Verification items for the finished model (mm, model axes). A direction names the side the tool comes from. Round coordinates to 2 decimals unless told otherwise and drop trailing zeros. Write each loop counter-clockwise with the first axis right and the second up, starting at its lowest first coordinate (ties: lowest second). Pieces come first, ordered by that corner, then holes. Notation, with made-up numbers: M 18.25,87 L 48.25,87 A20 cw 48.25,113 Z; hole C 11,62.5 d9. An arc over 180 degrees is marked long. One line per question, with ' | ' between items.
from build123d import *

# Parameters (mm, degrees)
SKETCH5_W           = 100
SKETCH5_H           = 170
BOSS_EXTRUDE2_DEPTH = 10
SKETCH7_W           = 20
SKETCH7_H           = 25
BOSS_EXTRUDE3_DEPTH = 25
SKETCH8_W           = 20
SKETCH8_H           = 25
BOSS_EXTRUDE4_DEPTH = 25
SKETCH11_R          = 5
CUT_EXTRUDE1_DEPTH  = 20
CUT_EXTRUDE2_START  = -20
SKETCH12_R          = 5
CUT_EXTRUDE2_DEPTH  = 20
SKETCH17_W          = 100
SKETCH17_H          = 10
BOSS_EXTRUDE6_DEPTH = 100


with BuildPart() as part:
    # Sketch5 → Boss-Extrude2 (new body)
    with BuildSketch(Plane(origin=(0, -50, 0), x_dir=(-1, 0, 0), z_dir=(0, -1, 0))):
        Rectangle(SKETCH5_W, SKETCH5_H)
    extrude(amount=-BOSS_EXTRUDE2_DEPTH)

    # Sketch7 → Boss-Extrude3 (add)
    with BuildSketch(Plane.ZY.offset(50)):
        with Locations((-75, -37.5)):
            Rectangle(SKETCH7_W, SKETCH7_H)
    extrude(amount=BOSS_EXTRUDE3_DEPTH)

    # Sketch8 → Boss-Extrude4 (add)
    with BuildSketch(Plane(origin=(50, 0, 0), x_dir=(0, 0, -1), z_dir=(1, 0, 0))):
        with Locations((75, -37.5)):
            Rectangle(SKETCH8_W, SKETCH8_H)
    extrude(amount=BOSS_EXTRUDE4_DEPTH)

    # Sketch11 → Cut-Extrude1 (cut)
    with BuildSketch(Plane.ZY.offset(75)):
        with Locations((-75, -40)):
            Circle(SKETCH11_R)
    extrude(amount=-CUT_EXTRUDE1_DEPTH, mode=Mode.SUBTRACT)

    # Sketch12 → Cut-Extrude2 (cut)
    with BuildSketch(Plane(origin=(75, 0, 0), x_dir=(0, 0, -1), z_dir=(1, 0, 0)).offset(CUT_EXTRUDE2_START)):
        with Locations(Location((75, -40, 0), (0, 0, 180))):
            Circle(SKETCH12_R)
    extrude(amount=CUT_EXTRUDE2_DEPTH, mode=Mode.SUBTRACT)

    # Sketch17 → Boss-Extrude6 (add)
    with BuildSketch(Plane.XY.offset(85)):
        with Locations((0, -45)):
            Rectangle(SKETCH17_W, SKETCH17_H)
    extrude(amount=BOSS_EXTRUDE6_DEPTH)


solid = part.part
1. Go/stop test with flat-tipped pins: P1, Ø7.5, axis at x = -61.5, y = -38, coming from the +Z side; P2, Ø3, axis at y = -44, z = 26.5, coming from the -X side; P3, Ø1.5, axis at x = -29.5, z = -31.5, coming from the +Y side. Record where each tip stops, or that it passes through.
Results:
P1: stops at z = -65 | P2: stops at x = -50 | P3: stops at y = -40
2. Section check A-A, the plane y = -31.25. Record the cut outline in (x, z), then the cut area to 3 significant figures.
Results:
outline: M -75,-85 L -50,-85 L -50,-65 L -75,-65 Z; M 50,-85 L 75,-85 L 75,-65 L 50,-65 Z | area: 1,000 mm2
3. Section check D-D, the plane z = -45. Record the cut outline in (x, y).
Results:
outline: M -50,-50 L 50,-50 L 50,-40 L -50,-40 Z
4. Thickness scan on line 1 (Z direction, x = 70.5, y = -40); line 2 (Y direction, x = -67.5, z = -75); line 3 (X direction, y = -42.75, z = 173.5). Record the ranges inside material, lowest first.
Results:
line 1: z = -85 to -80, -70 to -65 | line 2: y = -50 to -45, -35 to -25 | line 3: x = -50 to 50
5. Section check B-B, the plane z = -75. Record the cut outline in (x, y).
Results:
outline: M -75,-50 L 75,-50 L 75,-45 L 55,-45 L 55,-35 L 75,-35 L 75,-25 L 50,-25 L 50,-40 L -50,-40 L -50,-25 L -75,-25 L -75,-35 L -55,-35 L -55,-45 L -75,-45 Z
6. Tool access check on faces 1 (the face through (-65.14, -38.5, -70.23)), 2 (the face through (50, -45, 58)), 3 (the face through (50, -32, -75)), 4 (the face through (-50, -45, 58)). Record the directions out of +Z, -Z, +X, -X, +Y, -Y that give a thin tool (end or side, any length) a straight path to the whole face; none if there is none.
Results:
face 1: -X | face 2: +Z, +X, +Y, -Y | face 3: +Z, -Z, +Y | face 4: +Z, -X, +Y, -Y
7. Mould release check, pull along Y, two halves, no side actions. Record for faces 5 (the face through (62, -25, -75)), 6 (the face through (55, -40, -75)), 7 (the face through (62, -38, -65)): pulls with the +Y half, pulls with the -Y half, needs draft (parallel to the pull), parting line crosses it, or undercut.
Results:
face 5: pulls with the +Y half | face 6: undercut | face 7: needs draft
8. Section check C-C, the plane x = -8. Record the cut outline in (y, z), then the cut area to 3 significant figures.
Results:
outline: M -50,-85 L -40,-85 L -40,185 L -50,185 Z | area: 2,700 mm2
